from build123d import *

# Parameters (mm, degrees)
ESQUISSE1_W             = 68
ESQUISSE1_H             = 58
BOSS_EXTRU_1_DEPTH      = 3
BOSS_EXTRU_2_DEPTH      = 9
ESQUISSE4_W             = 3
ESQUISSE4_H             = 52
BOSS_EXTRU_3_DEPTH      = 65
ESQUISSE6_W             = 10
ESQUISSE6_H             = 3
BOSS_EXTRU_4_DEPTH      = 15
ESQUISSE7_R             = 1.6
ENL_V_MAT_EXTRU_1_DEPTH = 3
CONG_1_R                = 5


with BuildPart() as part:
    # Esquisse1 → Boss.-Extru.1 (new body)
    with BuildSketch(Plane.XY):
        Rectangle(ESQUISSE1_W, ESQUISSE1_H)
    extrude(amount=BOSS_EXTRU_1_DEPTH)

    # Esquisse2 → Boss.-Extru.2 (add)
    with BuildSketch(Plane.XY.offset(3)):
        Polygon((34, 26), (34, 29), (-34, 29), (-34, -29), (34, -29), (34, -26), (-31, -26), (-31, 26), align=None)
    extrude(amount=BOSS_EXTRU_2_DEPTH)

    # Esquisse4 → Boss.-Extru.3 (add)
    with BuildSketch(Plane(origin=(-31, 0, 0), x_dir=(0, 0, -1), z_dir=(1, 0, 0))):
        with Locations((-10.5, 0)):
            Rectangle(ESQUISSE4_W, ESQUISSE4_H)
    extrude(amount=BOSS_EXTRU_3_DEPTH)

    # Esquisse6 → Boss.-Extru.4 (add)
    with BuildSketch(Plane.XZ.offset(29)):
        with Locations((-29, 10.5)):
            Rectangle(ESQUISSE6_W, ESQUISSE6_H)
        with Locations((29, 10.5)):
            Rectangle(ESQUISSE6_W, ESQUISSE6_H)
    boss_extru_4 = extrude(amount=BOSS_EXTRU_4_DEPTH)

    # Esquisse7 → Enlèv. mat.-Extru.1 (cut)
    with BuildSketch(Plane.XY.offset(12)):
        with Locations((-29, -36.5)):
            Circle(ESQUISSE7_R)
        with Locations((29, -36.5)):
            Circle(ESQUISSE7_R)
    enl_v_mat_extru_1 = extrude(amount=-ENL_V_MAT_EXTRU_1_DEPTH, mode=Mode.SUBTRACT)

    # Symétrie1: Boss.-Extru.4, Enlèv. mat.-Extru.1 across plane
    add(boss_extru_4.mirror(Plane.ZX))
    add(enl_v_mat_extru_1.mirror(Plane.ZX), mode=Mode.SUBTRACT)

    # Congé1
    cong_1_edges = [part.edges().sort_by_distance(p)[0] for p in [
        (0, -29, 0),
        (-34, 0, 0),
        (0, 29, 0),
    ]]
    fillet(cong_1_edges, radius=CONG_1_R)


solid = part.part
Could you check a few things on this model? Use its own coordinates, in mm. A direction names the side the tool comes from. Give positions to 0.01 mm unless a question says otherwise; leave off trailing zeros. Order: outer loops, then holes, each group sorted by start corner. A loop starts at its lowest first (then second) coordinate and runs counter-clockwise, first axis right, second up.
1. We'd pull the mould along X, two halves only. Please class faces 5 (the cylindrical face through (0, -28, 2)), 6 (the flat face through (34, 1, 10)), 7 (the cylindrical face through (-29.35, 38.06, 10.52)): pulls with the +X half, pulls with the -X half, needs draft (parallel to the pull), parting line crosses it, or undercut.
2. Suppose I cut it at C-C (x = -10). List the corners of the cut face in (y, z) for me, plus the area to 3 significant figures.
3. Suppose I cut it at D-D (y = -17). List the corners of the cut face in (x, z) for me.
4. Will these pins go through, and if not, where does the flat tip stop? P1, Ø3.5, axis at x = 29, y = 36.5, coming from the -Z side; P2, Ø1.8, axis at x = -9.5, z = 4.5, coming from the +Y side; P3, Ø3, axis at x = -20.5, z = 4, coming from the -Y side.
5. Suppose I cut it at B-B (y = 36.5). List the corners of the cut face in (x, z) for me.
6. Suppose I cut it at A-A (x = 29). List the corners of the cut face in (y, z) for me.
7. For faces 1 (the flat face through (28.9, -34.7, 9)), 2 (the flat face through (-31, 0, 6)), 3 (the flat face through (-24, -36, 10)), 4 (the cylindrical face through (0, 27, 1)), which set-ups out of +Z, -Z, +X, -X, +Y, -Y let a thin tool reach every point of the face, with its end or its side?
8. I need wall thicknesses on L1, parallel to Y at x = -29, z = 10.8; L2, parallel to X at y = 36.5, z = 10; L3, parallel to Y at x = 10, z = 5. Which ranges of each line are inside material? Lowest first, please.
Solved:
1. face 5: needs draft
1. face 6: pulls with the +X half
1. face 7: undercut
2. outline: (-29, 5) arc R5 ccw to (-24, 0) - (24, 0) arc R5 ccw to (29, 5) - (29, 12) - (-29, 12) - close; hole (-26, 3) - (26, 3) - (26, 9) - (-26, 9) - close
2. area: 373 mm2
3. outline: (-34, 5) arc R5 ccw to (-29, 0) - (34, 0) - (34, 3) - (-31, 3) - (-31, 9) - (34, 9) - (34, 12) - (-34, 12) - close
4. P1: stops at z = 9
4. P2: stops at y = 29
4. P3: stops at y = -29
5. outline: (-34, 9) - (-30.6, 9) - (-30.6, 12) - (-34, 12) - close; (-27.4, 9) - (-24, 9) - (-24, 12) - (-27.4, 12) - close; (24, 9) - (27.4, 9) - (27.4, 12) - (24, 12) - close; (30.6, 9) - (34, 9) - (34, 12) - (30.6, 12) - close
6. outline: (-44, 9) - (-38.1, 9) - (-38.1, 12) - (-44, 12) - close; (-34.9, 9) - (-29, 9) - (-29, 5) arc R5 ccw to (-24, 0) - (24, 0) arc R5 ccw to (29, 5) - (29, 9) - (34.9, 9) - (34.9, 12) - (-34.9, 12) - close; (38.1, 9) - (44, 9) - (44, 12) - (38.1, 12) - close; hole (-26, 3) - (26, 3) - (26, 9) - (-26, 9) - close
7. face 1: -Z, +X, -X, -Y
7. face 2: +X
7. face 3: +Z, -Z, -Y
7. face 4: -Z, +X, -X, +Y
8. L1: y = -44 to -38.1, -34.9 to 34.9, 38.1 to 44
8. L2: x = -34 to -30.6, -27.4 to -24, 24 to 27.4, 30.6 to 34
8. L3: y = -29 to -26, 26 to 29
